Part model, mm, in its own coordinate system. A direction names the side the tool comes from. Give positions to 0.01 mm unless a question says otherwise; leave off trailing zeros. Write each loop counter-clockwise with the first axis right and the second up, starting at its lowest first coordinate (ties: lowest second). Pieces come first, ordered by that corner, then holes.
from build123d import *

# Parameters (mm, degrees)
SKETCH1_W           = 150
SKETCH1_H           = 70
BOSS_EXTRUDE1_DEPTH = 4.5
SKETCH2_W           = 50.3
SKETCH2_H           = 70.5
CUT_EXTRUDE1_DEPTH  = 166.590609637
CUT_EXTRUDE2_DEPTH  = 166.590609637
SKETCH4_R           = 1.65
CUT_EXTRUDE3_DEPTH  = 166.590609637
SKETCH5_R           = 3
CUT_EXTRUDE4_DEPTH  = 2
SKETCH7_W           = 4
SKETCH7_H           = 150
BOSS_EXTRUDE2_DEPTH = 4
SKETCH8_R           = 1.95
CUT_EXTRUDE5_DEPTH  = 10
SKETCH10_W          = 13
SKETCH10_H          = 45
CUT_EXTRUDE6_DEPTH  = 1


with BuildPart() as part:
    # Sketch1 → Boss-Extrude1 (new body)
    with BuildSketch(Plane(origin=(0, 0, 0), x_dir=(0, 1, 0), z_dir=(0, 0, 1))):
        with Locations((75, 35)):
            Rectangle(SKETCH1_W, SKETCH1_H)
    extrude(amount=BOSS_EXTRUDE1_DEPTH)

    # Sketch2 → Cut-Extrude1 (cut, through all)
    with BuildSketch(Plane(origin=(0, 0, 0), x_dir=(1, 0, 0), z_dir=(0, 0, -1))):
        with Locations((-38, -50)):
            Rectangle(SKETCH2_W, SKETCH2_H)
    extrude(amount=-CUT_EXTRUDE1_DEPTH, mode=Mode.SUBTRACT)

    # Sketch3 → Cut-Extrude2 (cut, through all)
    with BuildSketch(Plane.XY.offset(4.5)):
        with BuildLine():
            Line((-47.68869131, 108), (-47.68869131, 102))
            ThreePointArc((-47.68869131, 102), (-59.1, 105), (-47.68869131, 108))
        make_face()
        with BuildLine():
            Line((-47.68869131, 138), (-47.68869131, 132))
            ThreePointArc((-47.68869131, 132), (-59.1, 135), (-47.68869131, 138))
        make_face()
        with BuildLine():
            Line((-17.68869131, 138), (-17.68869131, 132))
            ThreePointArc((-17.68869131, 132), (-29.1, 135), (-17.68869131, 138))
        make_face()
        with BuildLine():
            Line((-17.68869131, 108), (-17.68869131, 102))
            ThreePointArc((-17.68869131, 102), (-29.1, 105), (-17.68869131, 108))
        make_face()
    extrude(amount=-CUT_EXTRUDE2_DEPTH, mode=Mode.SUBTRACT)

    # Sketch4 → Cut-Extrude3 (cut, through all)
    with BuildSketch(Plane.XY.offset(4.5)):
        with Locations((-59, 89.25)):
            Circle(SKETCH4_R)
        with Locations((-17, 89.25)):
            Circle(SKETCH4_R)
        with Locations((-17, 10.75)):
            Circle(SKETCH4_R)
        with Locations((-59, 10.75)):
            Circle(SKETCH4_R)
        with Locations((-66, 146)):
            Circle(SKETCH4_R)
        with Locations((-66, 4)):
            Circle(SKETCH4_R)
    extrude(amount=-CUT_EXTRUDE3_DEPTH, mode=Mode.SUBTRACT)

    # Sketch5 → Cut-Extrude4 (cut)
    with BuildSketch(Plane.XY.offset(4.5)):
        with Locations((-59, 89.25)):
            Circle(SKETCH5_R)
        with Locations((-17, 89.25)):
            Circle(SKETCH5_R)
        with Locations((-17, 10.75)):
            Circle(SKETCH5_R)
        with Locations((-59, 10.75)):
            Circle(SKETCH5_R)
        with Locations((-66, 146)):
            Circle(SKETCH5_R)
        with Locations((-66, 4)):
            Circle(SKETCH5_R)
    extrude(amount=-CUT_EXTRUDE4_DEPTH, mode=Mode.SUBTRACT)

    # Sketch7 → Boss-Extrude2 (add)
    with BuildSketch(Plane(origin=(0, 0, 0), x_dir=(1, 0, 0), z_dir=(0, 0, -1))):
        with Locations((-2, -75)):
            Rectangle(SKETCH7_W, SKETCH7_H)
    extrude(amount=BOSS_EXTRUDE2_DEPTH)

    # Sketch8 → Cut-Extrude5 (cut)
    with BuildSketch(Plane.YZ):
        with Locations(Location((15, 0.025, 0), (0, 0, 270))):
            Circle(SKETCH8_R)
        with Locations(Location((75, 0.125, 0), (0, 0, 270))):
            Circle(SKETCH8_R)
        with Locations(Location((135, 0.225, 0), (0, 0, 270))):
            Circle(SKETCH8_R)
    extrude(amount=-CUT_EXTRUDE5_DEPTH, mode=Mode.SUBTRACT)

    # Sketch10 → Cut-Extrude6 (cut)
    with BuildSketch(Plane(origin=(0, 0, 0), x_dir=(1, 0, 0), z_dir=(0, 0, -1))):
        with Locations((-38, -107.75)):
            Rectangle(SKETCH10_W, SKETCH10_H)
    extrude(amount=-CUT_EXTRUDE6_DEPTH, mode=Mode.SUBTRACT)


solid = part.part
1) Saw through at B-B (x = -53). Write the cut outline in (y, z).
Check result:
outline: (0, 0) - (14.75, 0) - (14.75, 4.5) - (0, 4.5) - close; (85.25, 0) - (98.9, 0) - (98.9, 4.5) - (85.25, 4.5) - close; (111.1, 0) - (128.9, 0) - (128.9, 4.5) - (111.1, 4.5) - close; (141.1, 0) - (150, 0) - (150, 4.5) - (141.1, 4.5) - close
2) Flat gauge pins, fed straight in: P1, Ø6.5, axis at x = -67, y = 146.5, coming from the +Z side; P2, Ø3, axis at y = 101, z = -3, coming from the -X side. Where does each tip first touch, or does it go through?
Check result:
P1: stops at z = 4.5
P2: stops at x = -4
3) Saw through at D-D (x = -36). Write the cut outline in (y, z), and give its area (3 significant figures).
Check result:
outline: (0, 0) - (14.75, 0) - (14.75, 4.5) - (0, 4.5) - close; (85.25, 1) - (130.25, 1) - (130.25, 0) - (150, 0) - (150, 4.5) - (85.25, 4.5) - close
area: 313 mm2
4) Saw through at A-A (y = 135). Write the cut outline in (x, z) (3 decimals), and give its area (3 significant figures).
Check result:
outline: (-70, 0) - (-59.1, 0) - (-59.1, 4.5) - (-70, 4.5) - close; (-47.689, 0) - (-29.1, 0) - (-29.1, 4.5) - (-47.689, 4.5) - close; (-17.689, 0) - (-10, 0) - (-10, 2.175) - (0, 2.175) - (0, 4.5) - (-17.689, 4.5) - close; (-4, -4) - (0, -4) - (0, -1.725) - (-4, -1.725) - close
area: 200 mm2
5) Saw through at C-C (y = 36). Write the cut outline in (x, z).
Check result:
outline: (-70, 0) - (-63.15, 0) - (-63.15, 4.5) - (-70, 4.5) - close; (-12.85, 0) - (-4, 0) - (-4, -4) - (0, -4) - (0, 4.5) - (-12.85, 4.5) - close
6) Mould opens along Z. For faces 1 (the cylindrical face through (-3.819, 135.086, 2.173)), 2 (the cylindrical face through (-17.65, 86.32, 3.51)), 3 (the flat face through (-64.7, 144.7, 2.5)) say: +Z half, -Z half, draft (parallel to the pull), parting line (faces both ways), or undercut.
Check result:
face 1: undercut
face 2: draft
face 3: +Z half
7) Drill centre lines: L1, parallel to X at y = 135, z = 1.6; L2, parallel to Y at x = -66, z = 1.4; L3, parallel to X at y = 35, z = 3. Where is each one in solid material? Low to high.
Check result:
L1: x = -70 to -59.1, -47.69 to -29.1, -17.69 to -10
L2: y = 0 to 2.35, 5.65 to 144.35, 147.65 to 150
L3: x = -70 to -63.15, -12.85 to 0
8) 3-axis set-ups, long thin cutter, end or side, ignore diameter. For faces 4 (the flat face through (-15.7, 88, 2.5)), 5 (the flat face through (-38, 85.25, 2)), 6 (the cylindrical face through (-3.819, 75.086, 2.073)): which of +Z, -Z, +X, -X, +Y, -Y reach the whole face in a straight line?
Check result:
face 4: +Z
face 5: +Z, -Z
face 6: +X
